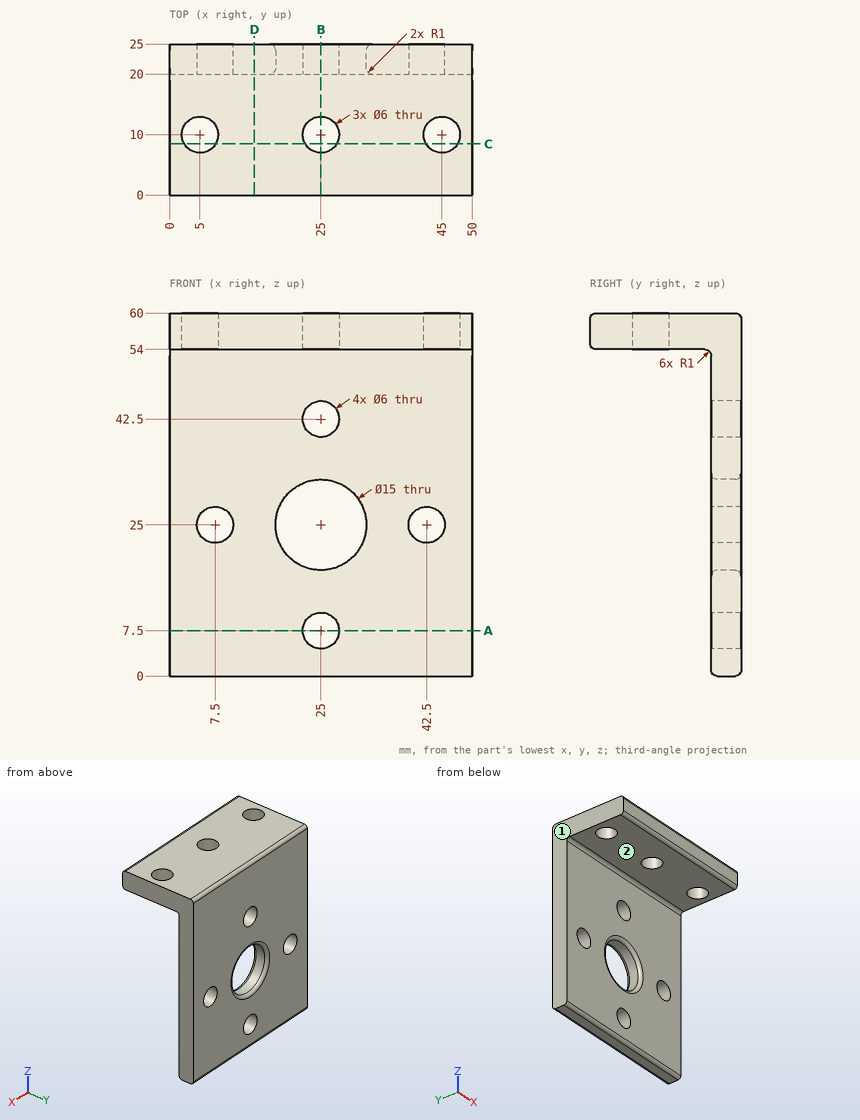
For this review, use the dimensioned drawing (mm, ordinates from the lowest corner) and the shaded views. A direction names the side the tool comes from. Round coordinates to 2 decimals unless told otherwise and drop trailing zeros. Order: outer loops, then holes, each group sorted by start corner. A loop starts at its lowest first (then second) coordinate and runs counter-clockwise, first axis right, second up. Notation, with made-up numbers: M -14.5,23.25 L 15.5,23.25 A10 ccw 15.5,39.25 Z; hole C 36.25,34 d5. An arc over 180 degrees is marked long. Use a Markdown table: item, result. Add a question column.
Item 1: Tool access review of the marked faces 1 and 2: name each direction out of +Z, -Z, +X, -X, +Y, -Y from which nothing blocks a thin tool from reaching the whole face with its end or side.
Item 2: Insertion check: pin 1 (9 mm diameter, centred on x = 15, y = 11.5, fed in from -Z); pin 2 (3 mm diameter, centred on x = 45, z = 45, fed in from -Y). Each pin has a flat end and moves straight along its axis. Give the tip position at first contact, or say it passes through.
Item 3: Add section A-A, the plane z = 7.5. Give the boundary of the cut face in (x, y).
Item 4: Add section D-D, the plane x = 14. Give the boundary of the cut face in (y, z), then the cut area to 3 significant figures.
Item 5: To check wall thickness, follow line 1 along Z through (x, y) = (25, 23.8); line 2 along X through (y, z) = (23.35, 42.5); line 3 along X through (y, z) = (20.5, 24.5). State the ranges of each line that lie inside material, in increasing order.
Item 6: Add section C-C, the plane y = 8.5. Give the boundary of the cut face in (x, z), then the cut area to 3 significant figures.
Item 7: Add section B-B, the plane x = 25. State how many separate pieces and enclosed holes the cut face has, then the cut area to 3 significant figures.
Geometry results:
| question | item | result |
|---|---|---|
| 1 | face 1 | +Z, -Z, -X, +Y, -Y |
| 1 | face 2 | -Z, +X, -X, -Y |
| 2 | pin 1 | stops at z = 54 |
| 2 | pin 2 | stops at y = 20 |
| 3 | outline | M 0,20 L 22,20 L 22,25 L 0,25 Z; M 28,20 L 50,20 L 50,25 L 28,25 Z |
| 4 | outline | M 0,55 A1 ccw 1,54 L 19,54 A1 cw 20,53 L 20,1 A1 ccw 21,0 L 24,0 A1 ccw 25,1 L 25,59 A1 ccw 24,60 L 1,60 A1 ccw 0,59 Z |
| 4 | area | 419 mm² |
| 5 | line 1 | z = 0 to 4.5, 10.5 to 17.5, 32.5 to 39.5, 45.5 to 60 |
| 5 | line 2 | x = 0 to 22, 28 to 50 |
| 5 | line 3 | x = 0 to 4.54, 10.46 to 17.38, 32.62 to 39.54, 45.46 to 50 |
| 6 | outline | M 0,54 L 2.4,54 L 2.4,60 L 0,60 Z; M 7.6,54 L 22.4,54 L 22.4,60 L 7.6,60 Z; M 27.6,54 L 42.4,54 L 42.4,60 L 27.6,60 Z; M 47.6,54 L 50,54 L 50,60 L 47.6,60 Z |
| 6 | area | 206 mm² |
| 7 | separate pieces | 5 |
| 7 | enclosed holes | 0 |
| 7 | area | 247 mm² |
